Model file for the job. Use its own axes, mm. A direction names the side the tool comes from. Coordinates: 2 decimals unless noted, no trailing zeros. Loops run counter-clockwise (first coordinate to the right, second up) from the corner with the lowest first, then second, coordinate; pieces in that order, holes last.
from build123d import *

# Parameters (mm, degrees)
SKETCH014_W             = 64.6
SKETCH014_H             = 86.556
PAD009_DEPTH            = 2
SKETCH015_W             = 64.6
SKETCH015_H             = 86.556
SKETCH015_W_2           = 62.6
SKETCH015_H_2           = 84.556
PAD010_DEPTH            = 5
SKETCH016_W             = 34
SKETCH016_H             = 1.5
PAD011_DEPTH            = 7.433333
SKETCH017_W             = 25
SKETCH017_H             = 15
PAD012_DEPTH            = 4.4
SKETCH018_R             = 2
POCKET005_DEPTH         = 2
SKETCH021_W             = 15
SKETCH021_H             = 5
PAD015_DEPTH            = 16.5
SKETCH022_W             = 4
SKETCH022_H             = 0.8
PAD016_DEPTH            = 17
BODY003_PLACEMENT_ANGLE = 180


with BuildPart() as part:
    # Sketch014 → Pad009 (new body)
    with BuildSketch(Plane.XY):
        Rectangle(SKETCH014_W, SKETCH014_H)
    extrude(amount=PAD009_DEPTH)

    # Sketch015 → Pad010 (join)
    with BuildSketch(Plane.XY):
        Rectangle(SKETCH015_W, SKETCH015_H)
        Rectangle(SKETCH015_W_2, SKETCH015_H_2, mode=Mode.SUBTRACT)
    extrude(amount=PAD010_DEPTH)

    # Sketch016 → Pad011 (join)
    with BuildSketch(Plane.XY):
        with Locations((0, 6.228)):
            Rectangle(SKETCH016_W, SKETCH016_H)
        with Locations((0, -31.228)):
            Rectangle(SKETCH016_W, SKETCH016_H)
    extrude(amount=PAD011_DEPTH)

    # Sketch017 → Pad012 (join)
    with BuildSketch(Plane.XY):
        with Locations((0, -12.5)):
            Rectangle(SKETCH017_W, SKETCH017_H)
    extrude(amount=PAD012_DEPTH)

    # Sketch018 → Pocket005 (cut)
    with BuildSketch(Plane.XY):
        with Locations((-26.5, 37.478)):
            Circle(SKETCH018_R)
        with Locations((-26.5, -37.478)):
            Circle(SKETCH018_R)
        with Locations((-26.5, 20.522)):
            Circle(SKETCH018_R)
        with Locations((26.5, 37.478)):
            Circle(SKETCH018_R)
        with Locations((26.5, 20.522)):
            Circle(SKETCH018_R)
        with Locations((26.5, -37.478)):
            Circle(SKETCH018_R)
    extrude(amount=POCKET005_DEPTH, mode=Mode.SUBTRACT)

    # Sketch021 → Pad015 (join)
    with BuildSketch(Plane.XY):
        with Locations((-7.5, -36.778)):
            Rectangle(SKETCH021_W, SKETCH021_H)
    extrude(amount=PAD015_DEPTH)

    # Sketch022 → Pad016 (join)
    with BuildSketch(Plane.XY):
        with Locations((-6, 39.278)):
            Rectangle(SKETCH022_W, SKETCH022_H)
        with Locations((6, 39.278)):
            Rectangle(SKETCH022_W, SKETCH022_H)
    extrude(amount=PAD016_DEPTH)


with BuildPart() as part_1:
    # Body003 placement: moved
    add(part.part.moved(Location((0, 0, 25.5))).rotate(Axis((0, 0, 25.5), (0, 1, 0)), BODY003_PLACEMENT_ANGLE))


solid = part_1.part
Q1. Slice it at D-D (x = 1). List the corners of the cut face in (y, z).
Answers:
outline: (-43.28, 20.5) - (-42.28, 20.5) - (-42.28, 23.5) - (-39.28, 23.5) - (-39.28, 9) - (-34.28, 9) - (-34.28, 23.5) - (-31.98, 23.5) - (-31.98, 18.07) - (-30.48, 18.07) - (-30.48, 23.5) - (-20, 23.5) - (-20, 21.1) - (-5, 21.1) - (-5, 23.5) - (5.48, 23.5) - (5.48, 18.07) - (6.98, 18.07) - (6.98, 23.5) - (42.28, 23.5) - (42.28, 20.5) - (43.28, 20.5) - (43.28, 25.5) - (-43.28, 25.5) - close
Q2. Slice it at B-B (z = 13.5). List the corners of the cut face in (x, y), and give its area (3 significant figures).
Answers:
outline: (-8, 38.88) - (-4, 38.88) - (-4, 39.68) - (-8, 39.68) - close; (0, -39.28) - (15, -39.28) - (15, -34.28) - (0, -34.28) - close; (4, 38.88) - (8, 38.88) - (8, 39.68) - (4, 39.68) - close
area: 81.4 mm2
Q3. Mould opens along X. For faces 3 (the flat face through (0, -43.278, 23)), 4 (the flat face through (-32.3, -1, 23)), 5 (the cylindrical face through (24.65, 19.76, 24.51)) say: +X half, -X half, draft (parallel to the pull), parting line (faces both ways), or undercut.
Answers:
face 3: draft
face 4: -X half
face 5: undercut
Q4. Which spindle directions (+Z, -Z, +X, -X, +Y, -Y) get a long thin tool onto all of the face, cutting with end or side? Do faces 1 (the cylindrical face through (-28.35, 19.76, 24.51)), 2 (the flat face through (-31.3, -1, 22)). Say none if no direction does.
Answers:
face 1: +Z, -Z
face 2: -Z
Q5. Drill centre lines: line 1 (X direction, y = -38.5, z = 21.75); line 2 (X direction, y = -17.5, z = 22.5); line 3 (Y direction, x = -3.5, z = 22). Where is each one in solid material? Low to high.
Answers:
line 1: x = -32.3 to -31.3, 0 to 15, 31.3 to 32.3
line 2: x = -32.3 to -31.3, -12.5 to 12.5, 31.3 to 32.3
line 3: y = -43.28 to -42.28, -31.98 to -30.48, -20 to -5, 5.48 to 6.98, 42.28 to 43.28
Q6. Slice it at A-A (x = -26.5). List the corners of the cut face in (y, z).
Answers:
outline: (-43.28, 20.5) - (-42.28, 20.5) - (-42.28, 23.5) - (-39.48, 23.5) - (-39.48, 25.5) - (-43.28, 25.5) - close; (-35.48, 23.5) - (18.52, 23.5) - (18.52, 25.5) - (-35.48, 25.5) - close; (22.52, 23.5) - (35.48, 23.5) - (35.48, 25.5) - (22.52, 25.5) - close; (39.48, 23.5) - (42.28, 23.5) - (42.28, 20.5) - (43.28, 20.5) - (43.28, 25.5) - (39.48, 25.5) - close
Q7. Flat gauge pins, fed straight in: P1, Ø3.5, axis at x = 26.5, y = -37.478, coming from the +Z side; P2, Ø12, axis at x = 1.5, y = -10, coming from the -Z side; P3, Ø10, axis at x = 1.5, z = 10.5, coming from the -Y side; P4, Ø0.8, axis at y = 6.5, z = 19.5, coming from the -X side. Where does each tip first touch, or does it go through?
Answers:
P1: passes through
P2: stops at z = 21.1
P3: stops at y = -39.28
P4: stops at x = -17
Q8. Slice it at C-C (y = -23.5). List the corners of the cut face in (x, z), and give its area (3 significant figures).
Answers:
outline: (-32.3, 20.5) - (-31.3, 20.5) - (-31.3, 23.5) - (31.3, 23.5) - (31.3, 20.5) - (32.3, 20.5) - (32.3, 25.5) - (-32.3, 25.5) - close
area: 135 mm2
